Source: CAD feature listing. Evaluate the final solid. Frame: model axes, mm. Face numbers are marked on the shaded views. Give positions to 0.01 mm unless a question says otherwise; leave off trailing zeros. Write each loop counter-clockwise with the first axis right and the second up, starting at its lowest first coordinate (ties: lowest second). Pieces come first, ordered by that corner, then holes. Notation, with made-up numbers: (31.25, 8.25) -> (82.25, 8.25) arc R33 ccw to (82.25, 36.25) -> close; hole circle Ø1 at (52, 58.5). An arc over 180 degrees is marked (long way). Use a Markdown table: item, result. Add a question column.
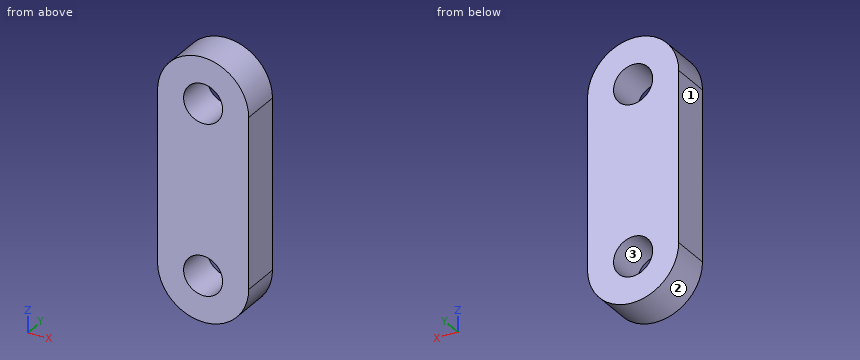
```python
from build123d import *

# Parameters (mm, degrees)
SKETCH1_R           = 1.5
BOSS_EXTRUDE1_DEPTH = 1.5


with BuildPart() as part:
    # Sketch1 → Boss-Extrude1 (new body, symmetric)
    with BuildSketch(Plane(origin=(0, 0, 0), x_dir=(1, 0, 0), z_dir=(0, 1, 0))):
        with BuildLine():
            Line((-3.5, -6.5), (-3.5, 6.5))
            ThreePointArc((-3.5, 6.5), (0, 10), (3.5, 6.5))
            Line((3.5, 6.5), (3.5, -6.5))
            ThreePointArc((3.5, -6.5), (0, -10), (-3.5, -6.5))
        make_face()
        with Locations((0, 6.5)):
            Circle(SKETCH1_R, mode=Mode.SUBTRACT)
        with Locations((0, -6.5)):
            Circle(SKETCH1_R, mode=Mode.SUBTRACT)
    extrude(amount=BOSS_EXTRUDE1_DEPTH, both=True)


solid = part.part
```
(1) Cut plane D-D on x = -1.25. Return the cut outline in (y, z), then the cut area to 3 significant figures.
(2) Mould query, pull axis X, two halves, no side actions, for the marked faces 1, 2 and 3. Classes: +X half, -X half, draft (parallel to the pull), parting line (faces both ways), or undercut.
(3) Cut plane A-A on x = 0. Return the cut outline in (y, z).
(4) Cut plane C-C on z = 7. Return the cut outline in (x, y), then the cut area to 3 significant figures.
(5) Cut plane B-B on y = 0.75. Return the cut outline in (x, z).
(6) Material intervals for L1, parallel to Z at x = 0, y = 0.8; L2, parallel to X at y = -0.4, z = -6.5; L3, parallel to Z at x = -1.25, y = 0.2, sorted ascending.
Output:
| question | item | result |
|---|---|---|
| 1 | outline | (-1.5, -9.77) -> (1.5, -9.77) -> (1.5, -7.33) -> (-1.5, -7.33) -> close; (-1.5, -5.67) -> (1.5, -5.67) -> (1.5, 5.67) -> (-1.5, 5.67) -> close; (-1.5, 7.33) -> (1.5, 7.33) -> (1.5, 9.77) -> (-1.5, 9.77) -> close |
| 1 | area | 48.7 mm^2 |
| 2 | face 1 | -X half |
| 2 | face 2 | parting line |
| 2 | face 3 | undercut |
| 3 | outline | (-1.5, -10) -> (1.5, -10) -> (1.5, -8) -> (-1.5, -8) -> close; (-1.5, -5) -> (1.5, -5) -> (1.5, 5) -> (-1.5, 5) -> close; (-1.5, 8) -> (1.5, 8) -> (1.5, 10) -> (-1.5, 10) -> close |
| 4 | outline | (-3.46, -1.5) -> (-1.41, -1.5) -> (-1.41, 1.5) -> (-3.46, 1.5) -> close; (1.41, -1.5) -> (3.46, -1.5) -> (3.46, 1.5) -> (1.41, 1.5) -> close |
| 4 | area | 12.3 mm^2 |
| 5 | outline | (-3.5, -6.5) arc R3.5 ccw to (3.5, -6.5) -> (3.5, 6.5) arc R3.5 ccw to (-3.5, 6.5) -> close; hole circle Ø3 at (0, -6.5); hole circle Ø3 at (0, 6.5) |
| 6 | L1 | -10 to -8, -5 to 5, 8 to 10 |
| 6 | L2 | -3.5 to -1.5, 1.5 to 3.5 |
| 6 | L3 | -9.77 to -7.33, -5.67 to 5.67, 7.33 to 9.77 |
